Input: part model. Units: mm. Frame: model coordinates. A direction names the side the tool comes from. Give positions to 0.01 mm unless a question says otherwise; leave off trailing zeros. Order: outer loops, then holes, each group sorted by start corner. A loop starts at its lowest first (then second) coordinate and runs counter-clockwise, first axis right, second up. Notation, with made-up numbers: (-12, 55.5) - (-4, 55.5) arc R21 ccw to (-4, 67.5) - close; hole circle Ø7 at (-40, 17). An arc over 180 degrees is marked (long way). Answer in a Markdown table with one row per item. Add a question column.
1. Access query for faces 5 (the face through (-12.939, -18.054, 20.66)), 6 (the face through (0, -138, 9)), 7 (the face through (1.565, -260.834, 11.957)). Directions: +Z, -Z, +X, -X, +Y, -Y. A direction counts if a zero-diameter tool reaches every point of the face in a straight line with its end or side. Return the directions, or none.
2. Mould query, pull axis Z, two halves, no side actions, for faces 1 (the face through (-10, -138, -3.175)), 2 (the face through (-10, -138, 19.05)), 3 (the face through (-21, -279.4, 10)), 4 (the face through (-10, -138, 22.225)). Classes: released by +Z, released by -Z, zero draft, split by the parting line, or undercut.
3. Section query A-A on y = -12.7. Return loops of the section in (x, z) (3 decimals), and give its area (3 significant figures).
4. Ray query, line 1 (Y direction, x = -10.25, z = -0.25); line 2 (Z direction, x = -17.75, y = -227) (3 decimals); line 3 (Z direction, x = 2.35, y = -266.7) (3 decimals). Return the intervals inside material, ascending. Write a range as [from, to].
5. Contact query for a flat-ended pin moving along its axis: pin 1 (10 mm diameter, centred on x = -9.525, y = -12.7, fed in from -Z). Output: stop coordinate, or through.
6. Section query B-B on x = -10.5. Return loops of the section in (y, z) (3 decimals), and give its area (3 significant figures).
7. Section query C-C on y = -266.7. Return loops of the section in (x, z) (3 decimals), and give its area (3 significant figures).
8. Section query D-D on z = 6.5. Return loops of the section in (x, y) (3 decimals).
```python
from build123d import *

# Parameters (mm, degrees)
F0_W     = 25.4
F0_H     = 25.4
F0_W_2   = 19.05
F0_H_2   = 19.05
F1_DEPTH = 279.4
F3_D     = 12.7
F3_DEPTH = 3.176
F5_D     = 12.7
F7_D     = 12.7
F7_DEPTH = 3.176


with BuildPart() as f1:
    # F0 (on Front) → F1 (new body)
    with BuildSketch(Plane.XZ):
        with Locations((-9.525, 9.525)):
            Rectangle(F0_W, F0_H)
        with Locations((-9.525, 9.525)):
            Rectangle(F0_W_2, F0_H_2, mode=Mode.SUBTRACT)
    extrude(amount=F1_DEPTH)

    # F3 (through all, one way)
    with BuildSketch(Plane.XY):
        with Locations((-9.525, -12.7)):
            Circle(F3_D / 2)
    extrude(amount=-F3_DEPTH, mode=Mode.SUBTRACT)

    # F5 (through all)
    with Locations(Plane(origin=(0, 0, 0), x_dir=(1, 0, 0), z_dir=(0, 0, -1))):
        with Locations((-9.525, 12.7)):
            Hole(F5_D / 2)

    # F7 (through all, one way)
    with BuildSketch(Plane(origin=(0, 0, 0), x_dir=(0, 1, 0), z_dir=(-1, 0, 0))):
        with Locations((-266.7, -9.525)):
            Circle(F7_D / 2)
    extrude(amount=-F7_DEPTH, mode=Mode.SUBTRACT)


solid = f1.part
```
Answer:
| question | item | result |
|---|---|---|
| 1 | face 5 | +Z, -Z |
| 1 | face 6 | +Y, -Y |
| 1 | face 7 | +X |
| 2 | face 1 | released by -Z |
| 2 | face 2 | undercut |
| 2 | face 3 | zero draft |
| 2 | face 4 | released by +Z |
| 3 | outline | (-22.225, -3.175) - (-15.875, -3.175) - (-15.875, 0) - (-19.05, 0) - (-19.05, 19.05) - (-15.875, 19.05) - (-15.875, 22.225) - (-22.225, 22.225) - close; (-3.175, -3.175) - (3.175, -3.175) - (3.175, 22.225) - (-3.175, 22.225) - (-3.175, 19.05) - (0, 19.05) - (0, 0) - (-3.175, 0) - close |
| 3 | area | 202 mm² |
| 4 | line 1 | y = [-279.4, -19.01], [-6.39, 0] |
| 4 | line 2 | z = [-3.175, 0], [19.05, 22.225] |
| 4 | line 3 | z = [-3.175, 3.175], [15.875, 22.225] |
| 5 | pin 1 | passes through |
| 6 | outline | (-279.4, -3.175) - (-18.975, -3.175) - (-18.975, 0) - (-279.4, 0) - close; (-279.4, 19.05) - (-18.975, 19.05) - (-18.975, 22.225) - (-279.4, 22.225) - close; (-6.425, -3.175) - (0, -3.175) - (0, 0) - (-6.425, 0) - close; (-6.425, 19.05) - (0, 19.05) - (0, 22.225) - (-6.425, 22.225) - close |
| 6 | area | 1,690 mm² |
| 7 | outline | (-22.225, -3.175) - (3.175, -3.175) - (3.175, 3.175) - (0, 3.175) - (0, 0) - (-19.05, 0) - (-19.05, 19.05) - (0, 19.05) - (0, 15.875) - (3.175, 15.875) - (3.175, 22.225) - (-22.225, 22.225) - close |
| 7 | area | 242 mm² |
| 8 | outline | (-22.225, -279.4) - (-19.05, -279.4) - (-19.05, 0) - (-22.225, 0) - close; (0, -279.4) - (3.175, -279.4) - (3.175, -272.283) - (0, -272.283) - close; (0, -261.117) - (3.175, -261.117) - (3.175, 0) - (0, 0) - close |
